For this review, take the finished solid that the model builds, in its own axes (mm). Face numbers are marked on the shaded views. A direction names the side the tool comes from. Give positions to 0.01 mm unless a question says otherwise; leave off trailing zeros. Order: outer loops, then holes, each group sorted by start corner. A loop starts at its lowest first (then second) coordinate and runs counter-clockwise, first axis right, second up.
from build123d import *

# Parameters (mm, degrees)
BOSS_EXTRUDE1_DEPTH      = 70
BOSS_EXTRUDE1_DEPTH_BACK = 30
SKETCH1_W                = 225
SKETCH1_H                = 150
CUT_EXTRUDE1_DEPTH       = 280.329554469
CUT_EXTRUDE2_DEPTH       = 68
CUT_EXTRUDE2_DEPTH_BACK  = 68
SKETCH8_R                = 19.05
CUT_EXTRUDE3_DEPTH       = 185
FILLET1_R                = 12
FILLET2_R                = 50.8
FILLET3_R                = 19.05
SKETCH13_W               = 7.4
SKETCH13_H               = 9.9
CUT_EXTRUDE4_DEPTH       = 4.318
FILLET4_R                = 0.635
FILLET4_OF_MIRROR2_R     = 0.635
SKETCH14_R               = 17.5254
CUT_EXTRUDE5_DEPTH       = 0.75
FILLET5_R                = 0.635
FILLET6_R                = 0.635
SKETCH16_W               = 15.1
SKETCH16_H               = 10.1
CUT_EXTRUDE6_DEPTH       = 3.05


with BuildPart() as part:
    # Sketch1 → Boss-Extrude1 (new, two sides: drawn at the far end of the back side and taken through both)
    with BuildSketch(Plane.XY.offset(-BOSS_EXTRUDE1_DEPTH_BACK)):
        with Locations((112.5, 75)):
            Rectangle(SKETCH1_W, SKETCH1_H)
    extrude(amount=BOSS_EXTRUDE1_DEPTH + BOSS_EXTRUDE1_DEPTH_BACK)

    # Sketch2 → Cut-Extrude1 (cut, through all)
    with BuildSketch(Plane.XZ):
        Polygon((225, 70), (171.371088333, 70), (225, 25), align=None)
        Polygon((0, 70), (15, 70), (0, 10), align=None)
    extrude(amount=-CUT_EXTRUDE1_DEPTH, mode=Mode.SUBTRACT)

    # Sketch7 → Cut-Extrude2 (cut, two sides: drawn at the far end of the back side and taken through both)
    with BuildSketch(Plane(origin=(0, 75, 0), x_dir=(1, 0, 0), z_dir=(0, 1, 0)).offset(-CUT_EXTRUDE2_DEPTH_BACK)):
        Polygon((215, 30.615528128), (215, -26.863959865), (169.551237162, -65), (18.903882032, -65), (5, -9.384471872), (5, 30.615528128), align=None)
    extrude(amount=CUT_EXTRUDE2_DEPTH + CUT_EXTRUDE2_DEPTH_BACK, mode=Mode.SUBTRACT)

    # Sketch8 → Cut-Extrude3 (cut)
    with BuildSketch(Plane.XZ):
        with Locations((40.375, -5)):
            Circle(SKETCH8_R)
        with BuildLine():
            Line((17.33584854, -30), (63.41415146, -30))
            ThreePointArc((63.41415146, -30), (55.439090064, -25.17113842), (56.02191035, -15.86631016))
            ThreePointArc((56.02191035, -15.86631016), (40.375, -24.05), (24.72808965, -15.86631016))
            ThreePointArc((24.72808965, -15.86631016), (25.310909936, -25.17113842), (17.33584854, -30))
        make_face()
        with Locations((184.625, -5)):
            Circle(SKETCH8_R)
        with BuildLine():
            ThreePointArc((200.27191035, -15.86631016), (184.625, -24.05), (168.97808965, -15.86631016))
            ThreePointArc((168.97808965, -15.86631016), (169.560909936, -25.17113842), (161.58584854, -30))
            Line((161.58584854, -30), (207.66415146, -30))
            ThreePointArc((207.66415146, -30), (199.689090064, -25.17113842), (200.27191035, -15.86631016))
        make_face()
    extrude(amount=-CUT_EXTRUDE3_DEPTH, mode=Mode.SUBTRACT)

    # Fillet1
    fillet1_edges = [part.edges().sort_by_distance(p)[0] for p in [
        (198.185544167, 0, 47.5),
        (225, 0, -2.5),
        (7.5, 0, 40),
        (93.185544167, 0, 70),
        (7.5, 150, 40),
        (93.185544167, 150, 70),
        (198.185544167, 150, 47.5),
        (225, 150, -2.5),
    ]]
    fillet(fillet1_edges, radius=FILLET1_R)

    # Fillet2
    # the kernel refuses this fillet: 50.8 mm, written as the material it takes off along each edge
    with BuildSketch(Plane(origin=(152.881400433, 150, 19.2), x_dir=(0, 0, 1), z_dir=(-1, 0, 0))) as fillet2_piece_1:
        with BuildLine():
            CenterArc((38.8, -12), 12, 0, 90)
            Line((50.8, -12), (50.8, 0))
            Line((50.8, 0), (38.8, 0))
        make_face()
    revolve(axis=Axis((152.881400433, 150, 19.2), (0, 1, 0)), revolution_arc=40, mode=Mode.SUBTRACT)
    with BuildSketch(Plane(origin=(152.881400433, 0, 19.2), x_dir=(0.6427876096865435, 0, 0.7660444431189747), z_dir=(0.7660444431189747, 0, -0.6427876096865435))) as fillet2_piece_2:
        with BuildLine():
            CenterArc((38.8, -12), 12, 0, 90)
            Line((50.8, -12), (50.8, 0))
            Line((50.8, 0), (38.8, 0))
        make_face()
    revolve(axis=Axis((152.881400433, 0, 19.2), (0, -1, 0)), revolution_arc=40, mode=Mode.SUBTRACT)
    with BuildSketch(Plane(origin=(171.371088333, 0, 70), x_dir=(-1, 0, 0), z_dir=(0, 1, 0))) as fillet2_piece_3:
        with BuildLine():
            CenterArc((FILLET2_R * 0.363970234266, -FILLET2_R), FILLET2_R, 90, 40)
            Line((-FILLET2_R * 0.27881737542, -FILLET2_R * 0.233955556881), (0, 0))
            Line((0, 0), (FILLET2_R * 0.363970234266, 0))
        make_face()
    extrude(amount=150, mode=Mode.SUBTRACT)

    # Fillet3
    # the kernel refuses this fillet: 19.05 mm, written as the material it takes off along each edge
    with BuildSketch(Plane(origin=(29.873790542, 150, 50.95), x_dir=(-0.9701425001453319, 0, 0.24253562503633305), z_dir=(-0.24253562503633305, 0, -0.9701425001453319))) as fillet3_piece_1:
        with BuildLine():
            CenterArc((7.05, -12), 12, 0, 90)
            Line((19.05, -12), (19.05, 0))
            Line((19.05, 0), (7.05, 0))
        make_face()
    fillet3_piece_1_solid = revolve(axis=Axis((29.873790542, 150, 50.95), (0, 1, 0)), revolution_arc=75.963756532, mode=Mode.PRIVATE)
    with BuildSketch(Plane(origin=(29.873790542, 0, 50.95), x_dir=(0, 0, 1), z_dir=(1, 0, 0))) as fillet3_piece_2:
        with BuildLine():
            CenterArc((7.05, -12), 12, 0, 90)
            Line((19.05, -12), (19.05, 0))
            Line((19.05, 0), (7.05, 0))
        make_face()
    fillet3_piece_2_solid = revolve(axis=Axis((29.873790542, 0, 50.95), (0, -1, 0)), revolution_arc=75.963756532, mode=Mode.PRIVATE)
    with BuildSketch(Plane(origin=(15, 0, 70), x_dir=(1, 0, 0), z_dir=(0, 1, 0))) as fillet3_piece_3:
        with BuildLine():
            CenterArc((FILLET3_R * 0.780776406404, FILLET3_R), FILLET3_R, 194.036243468, 75.963756532)
            Line((-FILLET3_R * 0.189366093741, FILLET3_R * 0.757464374964), (0, 0))
            Line((0, 0), (FILLET3_R * 0.780776406404, 0))
        make_face()
    fillet3_piece_3_solid = extrude(amount=150, mode=Mode.PRIVATE)
    add([fillet3_piece_1_solid, fillet3_piece_2_solid, fillet3_piece_3_solid], mode=Mode.SUBTRACT)

    # Sketch13 → Cut-Extrude4 (cut)
    with BuildSketch(Plane(origin=(225, 0, 0), x_dir=(0, 0, -1), z_dir=(1, 0, 0))):
        with Locations((-13.5, 43.25)):
            Rectangle(SKETCH13_W, SKETCH13_H)
    cut_extrude4 = extrude(amount=-CUT_EXTRUDE4_DEPTH, mode=Mode.SUBTRACT)

    # Fillet4
    fillet4_edges = [part.edges().sort_by_distance(p)[0] for p in [
        (220.682, 43.25, 9.8),
        (220.682, 38.3, 13.5),
        (220.682, 43.25, 17.2),
        (220.682, 48.2, 13.5),
        (225, 43.25, 9.8),
        (225, 48.2, 13.5),
        (225, 43.25, 17.2),
        (225, 38.3, 13.5),
    ]]
    fillet(fillet4_edges, radius=FILLET4_R)

    # Mirror2: Cut-Extrude4 across plane
    add(cut_extrude4.mirror(Plane.ZX.offset(75)), mode=Mode.SUBTRACT)

    # Fillet4 of Mirror2
    fillet4_of_mirror2_edges = [part.edges().sort_by_distance(p)[0] for p in [
        (220.682, 106.75, 9.8),
        (220.682, 111.7, 13.5),
        (220.682, 106.75, 17.2),
        (220.682, 101.8, 13.5),
        (225, 106.75, 9.8),
        (225, 101.8, 13.5),
        (225, 106.75, 17.2),
        (225, 111.7, 13.5),
    ]]
    fillet(fillet4_of_mirror2_edges, radius=FILLET4_OF_MIRROR2_R)

    # Sketch14 → Cut-Extrude5 (cut)
    with BuildSketch(Plane.XZ):
        with Locations(Location((147.32, 35, 0), (0, 0, 270))):
            Circle(SKETCH14_R)
    cut_extrude5 = extrude(amount=-CUT_EXTRUDE5_DEPTH, mode=Mode.SUBTRACT)

    # Fillet5
    fillet5_edges = [part.edges().sort_by_distance(p)[0] for p in [
        (147.32, 0, 52.5254),
    ]]
    fillet(fillet5_edges, radius=FILLET5_R)

    # Mirror4: Cut-Extrude5 across plane
    add(cut_extrude5.mirror(Plane.ZX.offset(75)), mode=Mode.SUBTRACT)

    # Fillet6
    fillet6_edges = [part.edges().sort_by_distance(p)[0] for p in [
        (147.32, 150, 52.5254),
    ]]
    fillet(fillet6_edges, radius=FILLET6_R)

    # Sketch16 → Cut-Extrude6 (cut)
    with BuildSketch(Plane(origin=(-2.352941176, 0, 0.588235294), x_dir=(0.24253562503633294, 0, 0.9701425001453319), z_dir=(-0.9701425001453319, 0, 0.24253562503633294))):
        with Locations((27.752024594, 112.5)):
            Rectangle(SKETCH16_W, SKETCH16_H)
    cut_extrude6 = extrude(amount=-CUT_EXTRUDE6_DEPTH, mode=Mode.SUBTRACT)

    # Mirror5: Cut-Extrude6 across plane
    add(cut_extrude6.mirror(Plane.ZX.offset(75)), mode=Mode.SUBTRACT)


solid = part.part
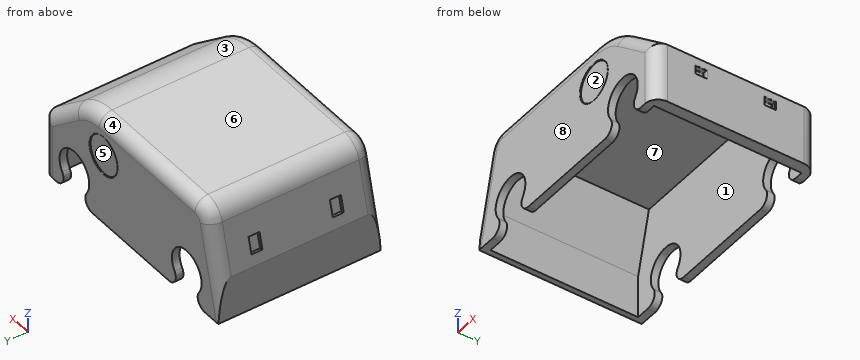
1) Draft analysis for pull direction Y (two halves, no side actions). For the marked faces 6, 7 and 8, state which applies: +Y half, -Y half, draft (parallel to the pull), parting line (faces both ways), or undercut.
Answer sheet:
face 6: draft
face 7: undercut
face 8: -Y half
2) We need section D-D on x = 147.32. Give the boundary of the cut face in (y, z) (3 decimals), then the cut area to 3 significant figures.
Answer sheet:
outline: (0, -30) - (7, -30) - (7, 65) - (143, 65) - (143, -30) - (150, -30) - (150, 16.84) arc R0.635 ccw to (149.365, 17.475) - (149.25, 17.475) - (149.25, 52.525) - (149.365, 52.525) arc R0.635 ccw to (150, 53.16) - (150, 58) arc R12 ccw to (138, 70) - (12, 70) arc R12 ccw to (0, 58) - (0, 53.16) arc R0.635 ccw to (0.635, 52.525) - (0.75, 52.525) - (0.75, 17.475) - (0.635, 17.475) arc R0.635 ccw to (0, 16.84) - close
area: 1,970 mm2
3) We need section B-B on x = 76.5. Give the boundary of the cut face in (y, z), then the cut area to 3 significant figures.
Answer sheet:
outline: (0, -30) - (7, -30) - (7, 65) - (143, 65) - (143, -30) - (150, -30) - (150, 58) arc R12 ccw to (138, 70) - (12, 70) arc R12 ccw to (0, 58) - close
area: 2,020 mm2
4) We need section A-A on y = 51.5. Give the boundary of the cut face in (x, z), then the cut area to 3 significant figures.
Answer sheet:
outline: (0, -30) - (5, -30) - (5, 9.38) - (18.9, 65) - (169.55, 65) - (215, 26.86) - (215, -30) - (225, -30) - (225, 25) - (185.54, 58.12) arc R50.8 ccw to (152.88, 70) - (29.87, 70) arc R19.05 ccw to (11.39, 55.57) - (0, 10) - close
area: 2,070 mm2
5) Clearance check with flat-ended pins moving along their axes: pin 1 (1 mm diameter, centred on y = 67.5, z = 38.5, fed in from +X); pin 2 (1.5 mm diameter, centred on x = 134.5, z = 40.5, fed in from +Y); pin 3 (5.5 mm diameter, centred on x = 4.5, z = 24.5, fed in from -Y). State where each tip first meets the part, or that it passes through.
Answer sheet:
pin 1: stops at x = 209.51
pin 2: stops at y = 149.25
pin 3: stops at y = 3.43
6) We need section C-C on z = -5. Count the separate pieces of the cut face and the enclosed holes in it, then the cut area to 3 significant figures.
Answer sheet:
separate pieces: 4
enclosed holes: 0
area: 4,040 mm2
7) Tool access review of the marked faces 1, 2, 3, 4 and 5: name each direction out of +Z, -Z, +X, -X, +Y, -Y from which nothing blocks a thin tool from reaching the whole face with its end or side.
Answer sheet:
face 1: -Z
face 2: -Y
face 3: +Z, +X, +Y, -Y
face 4: +Z, +X, -X, +Y
face 5: +Y
8) To check wall thickness, follow line 1 (X direction, y = 11, z = -17.5); line 2 (X direction, y = 3, z = -5) (3 decimals); line 3 (Y direction, x = 199, z = 24.5). State the ranges of each line that lie inside material, in increasing order.
Answer sheet:
line 1: x = 0 to 5, 215 to 224.96
line 2: x = 0.438 to 21.325, 59.425 to 165.575, 203.675 to 220.937
line 3: y = 0 to 7, 143 to 150
